The listing builds one solid part. Answer for the finished solid, in the listing's coordinates (mm). A direction names the side the tool comes from. Coordinates: 2 decimals unless noted, no trailing zeros. Write each loop counter-clockwise with the first axis right and the second up, starting at its lowest first coordinate (ties: lowest second). Pieces come first, ordered by that corner, then holes.
Autodesk Inventor part; units mm, degrees
ref_plane "BODY_N_XY" through (77, 0, 0) normal (0, 0, -1) x (1, 0, 0)
ref_plane "BODY_N_YZ" through (77, 0, 0) normal (1, 0, 0) x (0, -1, 0)
ref_plane "BODY_N_ZX" through (77, 0, 0) normal (0, -1, 0) x (0, 0, -1)
sketch "Sketch_8" plane through (0, 0, 0) normal (0, 0, 1) x (1, 0, 0)
  line L0 (0, 0) -> (-8, 0)
  line L1 (-8, 0) -> (-8, 4.3865)
  line L2 (-8, 4.3865) -> (-7.3865, 5)
  line L3 (-7.3865, 5) -> (0, 5)
  line L4 (0, 5) -> (0, 0)
  line L5 (0, 0) -> (-8, 0)
revolve "Revolution1" add sketch "Sketch_8" angle 360 about axis through (0, 0, 0) along (1, 0, 0)
thread "Thread1"
sketch "Sketch_9" plane through (0, 0, 0) normal (1, 0, 0) x (0, 0, -1)
  line L0 (-7.5, 4) -> (-7.5, -4)
  arc A0 (-7.5, -4) -> (-4, -7.5) centre (0, 0) ccw
  line L1 (-4, -7.5) -> (4, -7.5)
  arc A1 (4, -7.5) -> (7.5, -4) centre (0, 0) ccw
  line L2 (7.5, -4) -> (7.5, 4)
  arc A2 (7.5, 4) -> (4, 7.5) centre (0, 0) ccw
  line L3 (4, 7.5) -> (-4, 7.5)
  arc A3 (-4, 7.5) -> (-7.5, 4) centre (0, 0) ccw
extrude "Extrusion1" add sketch "Sketch_9" along normal blind 20.5
sketch "Sketch_6" plane through (20.5, 0, 0) normal (1, 0, 0) x (0, 0, -1)
  circle A0 centre (0, 0) radius 5.5
extrude "Extrusion2" add sketch "Sketch_6" along normal blind 39
sketch "Sketch_10" plane through (59.5, 0, 0) normal (1, 0, 0) x (0, 0, -1)
  line L0 (-6, 3.6056) -> (-6, -3.6056)
  arc A0 (-6, -3.6056) -> (-3.6056, -6) centre (0, 0) ccw
  line L1 (-3.6056, -6) -> (3.6056, -6)
  arc A1 (3.6056, -6) -> (6, -3.6056) centre (0, 0) ccw
  line L2 (6, -3.6056) -> (6, 3.6056)
  arc A2 (6, 3.6056) -> (3.6056, 6) centre (0, 0) ccw
  line L3 (3.6056, 6) -> (-3.6056, 6)
  arc A3 (-3.6056, 6) -> (-6, 3.6056) centre (0, 0) ccw
extrude "Extrusion3" add sketch "Sketch_10" along normal blind 9.5
sketch "Sketch7" plane through (0, 0, 0) normal (0, 0, 1) x (1, 0, 0)
  line L0 (5, 7.5) -> (5, 2.5)
  line L1 (5, 1.3066) -> (2.933, 2.5)
  line L2 (2.933, 2.5) -> (2.933, 7.067)
  line L3 (2.933, 7.067) -> (2.5, 7.5)
  line L4 (2.5, 7.5) -> (5, 7.5)
  line L5 (5, 7.5) -> (5, 1.3066)
revolve "Revolution2" cut sketch "Sketch7" angle 360 about axis through (5, 7.5, 0) along (0, 1, 0)
thread "Thread2"
sketch "Sketch_28" plane through (0, 0, 0) normal (0, 0, 1) x (1, 0, 0)
  line L0 (16, 7.5) -> (16, 2.5)
  line L1 (16, 1.3066) -> (13.933, 2.5)
  line L2 (13.933, 2.5) -> (13.933, 7.067)
  line L3 (13.933, 7.067) -> (13.5, 7.5)
  line L4 (13.5, 7.5) -> (16, 7.5)
  line L5 (16, 7.5) -> (16, 1.3066)
revolve "Revolution3" cut sketch "Sketch_28" angle 360 about axis through (16, 7.5, 0) along (0, 1, 0)
thread "Thread3"
sketch "Sketch8" plane through (0, 0, 0) normal (0, 0, 1) x (1, 0, 0)
  line L0 (69, 0) -> (64, 0)
  line L1 (62.8066, 0) -> (64, 2.067)
  line L2 (64, 2.067) -> (68.567, 2.067)
  line L3 (68.567, 2.067) -> (69, 2.5)
  line L4 (69, 2.5) -> (69, 0)
  line L5 (69, 0) -> (62.8066, 0)
revolve "Revolution4" cut sketch "Sketch8" angle 360 about axis through (69, 0, 0) along (1, 0, 0)
thread "Thread4"
sketch "Sketch_16" plane through (0, 0, 0) normal (0, 0, 1) x (1, 0, 0)
  line L0 (40.5, 0) -> (-8, 0)
  line L1 (-8, 0) -> (-8, 2)
  line L2 (-8, 2) -> (20.5, 2)
  line L3 (20.5, 2) -> (20.5, 5)
  line L4 (20.5, 5) -> (40.5, 5)
  line L5 (40.5, 5) -> (40.5, 0)
  line L6 (40.5, 0) -> (-8, 0)
revolve "Revolution5" cut sketch "Sketch_16" angle 360 about axis through (40.5, 0, 0) along (1, 0, 0)
ref_plane "BODY_N_XY" through (77, 0, 0) normal (0, 0, -1) x (1, 0, 0)
ref_plane "BODY_N_YZ" through (77, 0, 0) normal (1, 0, 0) x (0, -1, 0)
ref_plane "BODY_N_ZX" through (77, 0, 0) normal (0, -1, 0) x (0, 0, -1)
ref_plane "NUT2_XY" through (69, 0, 0) normal (1, 0, 0) x (0, 0, -1)
ref_plane "NUT2_YZ" through (69, 0, 0) normal (0, 0, -1) x (0, 1, 0)
ref_plane "NUT2_ZX" through (69, 0, 0) normal (0, 1, 0) x (1, 0, 0)
ref_plane "SW1_XY" through (25, 0, 0) normal (1, 0, 0) x (0, 0, -1)
ref_plane "SW1_YZ" through (25, 0, 0) normal (0, 0, -1) x (0, 1, 0)
ref_plane "SW1_ZX" through (25, 0, 0) normal (0, 1, 0) x (1, 0, 0)
ref_plane "SW2_XY" through (55, 0, 0) normal (-1, 0, 0) x (0, 0, -1)
ref_plane "SW2_YZ" through (55, 0, 0) normal (0, 0, -1) x (0, -1, 0)
ref_plane "SW2_ZX" through (55, 0, 0) normal (0, -1, 0) x (-1, 0, 0)
ref_plane "SW_R1_XY" through (25, -12.5, 0) normal (1, 0, 0) x (0, 0, -1)
ref_plane "SW_R1_YZ" through (25, -12.5, 0) normal (0, 0, -1) x (0, 1, 0)
ref_plane "SW_R1_ZX" through (25, -12.5, 0) normal (0, 1, 0) x (1, 0, 0)
ref_plane "SW_R2_XY" through (55, -12.5, 0) normal (-1, 0, 0) x (0, 0, -1)
ref_plane "SW_R2_YZ" through (55, -12.5, 0) normal (0, 0, -1) x (0, -1, 0)
ref_plane "SW_R2_ZX" through (55, -12.5, 0) normal (0, -1, 0) x (-1, 0, 0)
ref_plane "body_XY" through (0, 0, 0) normal (1, 0, 0) x (0, 0, -1)
ref_plane "body_YZ" through (0, 0, 0) normal (0, 0, -1) x (0, 1, 0)
ref_plane "body_ZX" through (0, 0, 0) normal (0, 1, 0) x (1, 0, 0)
properties part number "10-CJ2B10-15RZ(1_0)_BODY"
Q1. Determine the mould class of faces 5 (the face through (6, -2, 0)), 6 (the face through (0, 5, 2)), 7 (the face through (64, -6, 0)) for opening direction Y: released by +Y, released by -Y, zero draft, split by the parting line, or undercut.
Answers below:
face 5: undercut
face 6: zero draft
face 7: released by -Y
Q2. The part is cut by section B-B, the plane x = 5. Write down the section's boundary in (y, z), then the cut area to 3 significant figures.
Answers below:
outline: (-7.5, -4) arc R8.5 ccw to (-4, -7.5) - (4, -7.5) arc R8.5 ccw to (7.5, -4) - (7.5, -2.5) - (7.07, -2.07) - (2.5, -2.07) - (1.8, -0.86) arc R2 cw (long way) to (1.8, 0.86) - (2.5, 2.07) - (7.07, 2.07) - (7.5, 2.5) - (7.5, 4) arc R8.5 ccw to (4, 7.5) - (-4, 7.5) arc R8.5 ccw to (-7.5, 4) - close
area: 170 mm2
Q3. Given pin 1 (3 mm diameter, centred on y = 6, z = -0.5, fed in from -X); pin 2 (6 mm diameter, centred on x = 64.5, y = -1, fed in from +Z); pin 3 (3 mm diameter, centred on y = 0, z = 0, fed in from -X), each flat-ended and moving along its own axis, determine where each tip first touches the part or whether it passes through.
Answers below:
pin 1: stops at x = -7.87
pin 2: stops at z = 6
pin 3: stops at x = 40.5
Q4. Find the intervals of material crossed by probe 1 along X at (y, z) = (-5.25, 4.25); probe 2 along X at (y, z) = (-4, 1); probe 3 along X at (y, z) = (5.5, 1.5), in increasing order.
Answers below:
probe 1: x = 0 to 20.5, 59.5 to 69
probe 2: x = -8 to 20.5, 40.5 to 69
probe 3: x = 0 to 3.58, 6.42 to 14.58, 17.42 to 20.5, 59.5 to 69
Q5. The part is cut by section A-A, the plane x = 39. Write down the section's boundary in (y, z).
Answers below:
outline: circle Ø11 at (0, 0); hole circle Ø10 at (0, 0)
Q6. Which of the six approach directions +Z, -Z, +X, -X, +Y, -Y give full straight-line access (tool end or side, diameter ignored) to faces 1 (the face through (64.2, 4.9, 5)), 2 (the face through (64, 0, 6)), 3 (the face through (40.5, 0, 0)), 4 (the face through (64, 6, 0))?
Answers below:
face 1: +Z, +X, +Y
face 2: +Z, +X, +Y, -Y
face 3: none
face 4: +Z, -Z, +X, +Y
